Verification items for the finished model (mm, model axes). A direction names the side the tool comes from. Round coordinates to 2 decimals unless told otherwise and drop trailing zeros. Order: outer loops, then holes, each group sorted by start corner. A loop starts at its lowest first (then second) coordinate and runs counter-clockwise, first axis right, second up. Notation, with made-up numbers: (-27.5, 41) -> (24.5, 41) arc R29 ccw to (24.5, 64) -> close; hole circle Ø10 at (35.25, 36). An arc over 180 degrees is marked (long way). Put each result on its own line as item: value.
```python
from build123d import *

# Parameters (mm, degrees)
BOSS_EXTRUDE4_DEPTH                              = 12.7
SKETCH10_W                                       = 76.2
SKETCH10_H                                       = 6.35
BOSS_EXTRUDE5_DEPTH                              = 6.35
CSK_FOR_1_4_FLAT_HEAD_MACHINE_SCREW1_D           = 6.7564
CSK_FOR_1_4_FLAT_HEAD_MACHINE_SCREW1_CSINK_D     = 12.8778
CSK_FOR_1_4_FLAT_HEAD_MACHINE_SCREW1_CSINK_ANGLE = 82
BOSS_EXTRUDE6_DEPTH                              = 7.62
FILLET1_R                                        = 12.7
SKETCH20_R                                       = 15.875
SKETCH20_R_2                                     = 6.35
BOSS_EXTRUDE7_DEPTH                              = 12.7
BOSS_EXTRUDE8_DEPTH                              = 6.35


with BuildPart() as part:
    # Sketch1 → Boss-Extrude4 (new body)
    with BuildSketch(Plane(origin=(0, 0, 0), x_dir=(1, 0, 0), z_dir=(0, 1, 0))):
        with BuildLine():
            Line((-25.4, 17.4625), (25.4, 17.4625))
            ThreePointArc((25.4, 17.4625), (34.380256121, 13.742756121), (38.1, 4.7625))
            Line((38.1, 4.7625), (38.1, -11.1125))
            Line((38.1, -11.1125), (-38.1, -11.1125))
            Line((-38.1, -11.1125), (-38.1, 4.7625))
            ThreePointArc((-38.1, 4.7625), (-34.380256121, 13.742756121), (-25.4, 17.4625))
        make_face()
    extrude(amount=BOSS_EXTRUDE4_DEPTH)

    # Sketch10 → Boss-Extrude5 (add)
    with BuildSketch(Plane(origin=(0, 0, 0), x_dir=(1, 0, 0), z_dir=(0, 1, 0))):
        with Locations((0, -14.2875)):
            Rectangle(SKETCH10_W, SKETCH10_H)
    extrude(amount=BOSS_EXTRUDE5_DEPTH)

    # CSK for 1/4 Flat Head Machine Screw1 (through all)
    with Locations(Plane(origin=(0, 12.7, 0), x_dir=(1, 0, 0), z_dir=(0, 1, 0))):
        with Locations((-25.4, 4.7625), (25.4, 4.7625)):
            CounterSinkHole(CSK_FOR_1_4_FLAT_HEAD_MACHINE_SCREW1_D / 2, CSK_FOR_1_4_FLAT_HEAD_MACHINE_SCREW1_CSINK_D / 2, counter_sink_angle=CSK_FOR_1_4_FLAT_HEAD_MACHINE_SCREW1_CSINK_ANGLE)

    # Sketch19 → Boss-Extrude6 (add)
    with BuildSketch(Plane.XY.offset(11.1125)):
        with BuildLine():
            Line((-15.875, 12.7), (15.875, 12.7))
            Line((15.875, 12.7), (15.875, 63.5))
            ThreePointArc((15.875, 63.5), (0, 47.625), (-15.875, 63.5))
            Line((-15.875, 63.5), (-15.875, 12.7))
        make_face()
    extrude(amount=-BOSS_EXTRUDE6_DEPTH)

    # Fillet1
    fillet1_edges = [part.edges().sort_by_distance(p)[0] for p in [
        (-15.875, 12.7, 7.3025),
        (15.875, 12.7, 7.3025),
    ]]
    fillet(fillet1_edges, radius=FILLET1_R)

    # Sketch20 → Boss-Extrude7 (add)
    with BuildSketch(Plane(origin=(0, 0, 3.4925), x_dir=(-1, 0, 0), z_dir=(0, 0, -1))):
        with Locations((0, 63.5)):
            Circle(SKETCH20_R)
        with Locations((0, 63.5)):
            Circle(SKETCH20_R_2, mode=Mode.SUBTRACT)
    extrude(amount=-BOSS_EXTRUDE7_DEPTH)

    # Sketch21 → Boss-Extrude8 (add, symmetric)
    with BuildSketch(Plane(origin=(0, 0, 0), x_dir=(0, 0, -1), z_dir=(1, 0, 0))):
        Polygon((-3.4925, 57.15), (17.4625, 12.7), (-3.4925, 12.7), align=None)
    extrude(amount=BOSS_EXTRUDE8_DEPTH, both=True)


solid = part.part
```
Item 1: Sectioned sample at A-A, the plane z = 6.5. Record the boundary of the cut face in (x, y) (3 decimals).
Geometry check:
outline: (-38.1, 0) -> (38.1, 0) -> (38.1, 12.7) -> (28.575, 12.7) arc R12.7 cw to (15.875, 25.4) -> (15.875, 63.5) arc R15.875 ccw to (-15.875, 63.5) -> (-15.875, 25.4) arc R12.7 cw to (-28.575, 12.7) -> (-38.1, 12.7) -> close; hole circle Ø12.7 at (0, 63.5)
Item 2: Tool access check on faces 4 (the face through (6.35, 25, -2)), 5 (the face through (-18, 12.7, -3)), 6 (the face through (-15.875, 45, 7)). Record the directions out of +Z, -Z, +X, -X, +Y, -Y that give a thin tool (end or side, any length) a straight path to the whole face; none if there is none.
Geometry check:
face 4: -Z, +X, +Y
face 5: -Z, -X, +Y
face 6: +Z, -Z, -X, +Y
Item 3: Sectioned sample at D-D, the plane x = 11. Record the boundary of the cut face in (y, z), then the cut area to 3 significant figures.
Geometry check:
outline: (0, -17.46) -> (12.7, -17.46) -> (12.7, 3.49) -> (74.95, 3.49) -> (74.95, 16.19) -> (52.05, 16.19) -> (52.05, 11.11) -> (6.35, 11.11) -> (6.35, 17.46) -> (0, 17.46) -> close
area: 994 mm2
Item 4: Release check for a two-part mould opening along Y. For faces 1 (the face through (38.1, 6, 4)), 2 (the face through (0, 24, 11.112)), 3 (the face through (-22.6, 9.35, -2.62)) record: pulls with the +Y half, pulls with the -Y half, needs draft (parallel to the pull), parting line crosses it, or undercut.
Geometry check:
face 1: needs draft
face 2: undercut
face 3: pulls with the +Y half
Item 5: Sectioned sample at B-B, the plane y = 59. Record the boundary of the cut face in (x, z) (1 decimal), then the cut area to 3 significant figures.
Geometry check:
outline: (-15.9, 3.5) -> (-4.5, 3.5) -> (-4.5, 16.2) -> (-15.2, 16.2) -> (-15.2, 11.1) -> (-15.9, 11.1) -> close; (4.5, 3.5) -> (15.9, 3.5) -> (15.9, 11.1) -> (15.2, 11.1) -> (15.2, 16.2) -> (4.5, 16.2) -> close
area: 283 mm2
Item 6: Depth check by flat-ended pin: pin 1 Ø17 at (x, y) = (-16.5, 49) entering from +Z; pin 2 Ø1 at (x, y) = (-11, 46.5) entering from -Z; pin 3 Ø6 at (y, z) = (38, 7.5) entering from +X (3 decimals). Enter the tip coordinate at first touch or a pass-through.
Geometry check:
pin 1: z = 16.19
pin 2: z = 3.49
pin 3: x = 15.875
Item 7: Material ranges on line 1 along Y through (x, z) = (0, 12.25) (3 decimals); line 2 along Z through (x, y) = (25.4, 5.75); line 3 along X through (y, z) = (63.5, 12) (3 decimals), recorded low to high.
Geometry check:
line 1: 0 to 6.35, 47.625 to 57.15, 69.85 to 79.375
line 2: -17.46 to -8.14, -1.38 to 17.46
line 3: -15.875 to -6.35, 6.35 to 15.875
